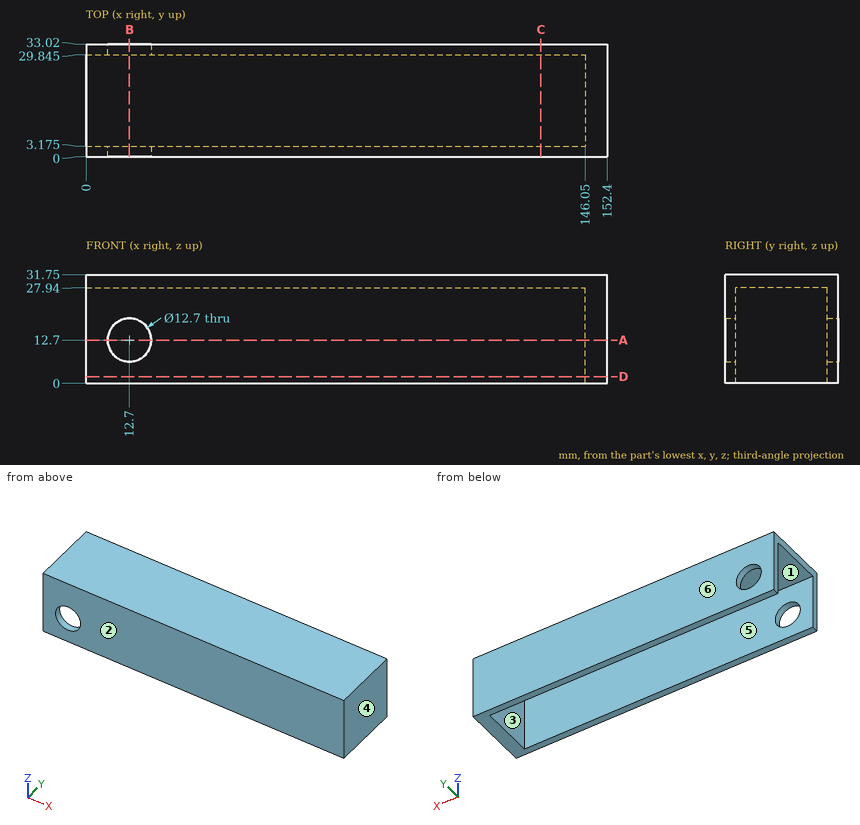
The drawing under review shows one solid part. Ordinate dimensions are in mm from its lowest x, y, z. A direction names the side the tool comes from. Give positions to 0.01 mm unless a question says otherwise; leave off trailing zeros. Loops run counter-clockwise (first coordinate to the right, second up) from the corner with the lowest first, then second, coordinate; pieces in that order, holes last. Notation, with made-up numbers: M 44.5,0 L 66.5,0 A33 cw 66.5,34 Z; hole C 77.25,46 d9. An arc over 180 degrees is marked long. Return JSON: item names as keys, results as strings. Group by question number.
Item 1: For probe 1 along Y at (x, z) = (62, 2) (3 decimals); probe 2 along Z at (x, y) = (12.7, 2.25); probe 3 along X at (y, z) = (31.3, 12.7), list the stretches that pass through material, from the lowest coordinate up.
Item 2: We need section C-C (x = 133). Give the boundary of the cut face in (y, z) (3 decimals).
Item 3: We need section D-D (z = 2). Give the boundary of the cut face in (x, y) (3 decimals).
Item 4: Mouldability with a two-part tool opening along Y and no side actions: class the marked faces 3, 4, 5 and 6 as released by +Y, released by -Y, zero draft, split by the parting line, or undercut.
Item 5: We need section B-B (x = 12.7). Give the boundary of the cut face in (y, z) (3 decimals).
Item 6: We need section A-A (z = 12.7). Give the boundary of the cut face in (x, y) (3 decimals), and give its area (3 significant figures).
Item 7: Insertion check: pin 1 Ø6 at (x, z) = (121, 5) entering from -Y; pin 2 Ø8 at (x, y) = (87.5, 15.5) entering from -Z; pin 3 Ø11.5 at (x, z) = (12.7, 12.7) entering from -Y; pin 4 Ø5 at (y, z) = (8, 7) entering from -X. Each pin has a flat end and moves straight along its axis. Give the tip position at first contact, or say it passes through.
Item 8: Tool access review of the marked faces 1 and 2: name each direction out of +Z, -Z, +X, -X, +Y, -Y from which nothing blocks a thin tool from reaching the whole face with its end or side.
Output:
{
 "1": {"probe 1": "y = 0 to 3.175, 29.845 to 33.02", "probe 2": "z = 0 to 6.35, 19.05 to 31.75", "probe 3": "x = 0 to 6.35, 19.05 to 152.4"},
 "2": {"outline": "M 0,0 L 3.175,0 L 3.175,27.94 L 29.845,27.94 L 29.845,0 L 33.02,0 L 33.02,31.75 L 0,31.75 Z"},
 "3": {"outline": "M 0,0 L 152.4,0 L 152.4,33.02 L 0,33.02 L 0,29.845 L 146.05,29.845 L 146.05,3.175 L 0,3.175 Z"},
 "4": {"face 3": "undercut", "face 4": "zero draft", "face 5": "undercut", "face 6": "released by +Y"},
 "5": {"outline": "M 0,0 L 3.175,0 L 3.175,6.35 L 0,6.35 Z; M 0,19.05 L 3.175,19.05 L 3.175,27.94 L 29.845,27.94 L 29.845,19.05 L 33.02,19.05 L 33.02,31.75 L 0,31.75 Z; M 29.845,0 L 33.02,0 L 33.02,6.35 L 29.845,6.35 Z"},
 "6": {"outline": "M 0,0 L 6.35,0 L 6.35,3.175 L 0,3.175 Z; M 0,29.845 L 6.35,29.845 L 6.35,33.02 L 0,33.02 Z; M 19.05,0 L 152.4,0 L 152.4,33.02 L 19.05,33.02 L 19.05,29.845 L 146.05,29.845 L 146.05,3.175 L 19.05,3.175 Z", "area": "1,060 mm^2"},
 "7": {"pin 1": "stops at y = 0", "pin 2": "stops at z = 27.94", "pin 3": "passes through", "pin 4": "stops at x = 146.05"},
 "8": {"face 1": "-Z, -X", "face 2": "+Z, -Z, +X, -X, -Y"}
}
